```python
from build123d import *

# Parameters (mm, degrees)
SKETCH1_W           = 1000
SKETCH1_H           = 500
BOSS_EXTRUDE1_DEPTH = 400
SKETCH2_R           = 150
BOSS_EXTRUDE2_DEPTH = 150


with BuildPart() as part:
    # Sketch1 → Boss-Extrude1 (new body)
    with BuildSketch(Plane(origin=(0, 0, 0), x_dir=(1, 0, 0), z_dir=(0, 1, 0))):
        Polygon((1400, -200), (1000, 0), (1000, 500), (1400, 700), align=None)
        with Locations((500, 250)):
            Rectangle(SKETCH1_W, SKETCH1_H)
    extrude(amount=BOSS_EXTRUDE1_DEPTH)

    # Sketch2 → Boss-Extrude2 (add)
    with BuildSketch(Plane(origin=(0, 400, 0), x_dir=(1, 0, 0), z_dir=(0, 1, 0))):
        with Locations(Location((500, 250, 0), (0, 0, 270))):
            Circle(SKETCH2_R)
    extrude(amount=BOSS_EXTRUDE2_DEPTH)


solid = part.part
```
Source: CAD feature listing. Evaluate the final solid. Frame: model axes, mm. A direction names the side the tool comes from. Round coordinates to 2 decimals unless told otherwise and drop trailing zeros. Order: outer loops, then holes, each group sorted by start corner. A loop starts at its lowest first (then second) coordinate and runs counter-clockwise, first axis right, second up. Notation, with made-up numbers: (30, 6) -> (45, 6) arc R8 cw to (45, 10) -> close; hole circle Ø4 at (0, -34). An arc over 180 degrees is marked (long way). Use CSV: the item, a comma, the result in double quotes.
(1) Section C-C on y = 137.5. Return the cut outline in (x, z).
Report:
outline,"(0, -500) -> (1000, -500) -> (1400, -700) -> (1400, 200) -> (1000, 0) -> (0, 0) -> close"
(2) Section A-A on z = -250. Return the cut outline in (x, y).
Report:
outline,"(0, 0) -> (1400, 0) -> (1400, 400) -> (650, 400) -> (650, 550) -> (350, 550) -> (350, 400) -> (0, 400) -> close"
(3) Access query for faces 1 (the face through (710, 0, -256)), 2 (the face through (493, 197, 0)), 3 (the face through (493, 197, -500)), 4 (the face through (502, 550, -252)), 5 (the face through (545.06, 473.95, -106.93)). Directions: +Z, -Z, +X, -X, +Y, -Y. A direction counts if a zero-diameter tool reaches every point of the face in a straight line with its end or side. Return the directions, or none.
Report:
face 1,"+Z, -Z, +X, -X, -Y"
face 2,"+Z, -X, +Y, -Y"
face 3,"-Z, -X, +Y, -Y"
face 4,"+Z, -Z, +X, -X, +Y"
face 5,"+Y"
(4) Ray query, L1, parallel to Z at x = 220.5, y = 146; L2, parallel to Y at x = 222.5, z = -35.5; L3, parallel to X at y = 119, z = 150.5. Return the intervals inside material, ascending.
Report:
L1,"-500 to 0"
L2,"0 to 400"
L3,"1301 to 1400"
(5) Section D-D on z = -593.5. Return the cut outline in (x, y), and give its area (3 significant figures).
Report:
outline,"(1187, 0) -> (1400, 0) -> (1400, 400) -> (1187, 400) -> close"
area,"85,200 mm^2"
(6) First-contact query: pin 1 Ø4 at (x, y) = (620, 127) entering from +Z; pin 2 Ø2 at (x, z) = (912.5, -449) entering from +Y; pin 3 Ø10 at (x, y) = (435.5, 296.5) entering from -Z. Flat tips, straight axial feed; report the tip coordinate or a pass-through.
Report:
pin 1,"z = 0"
pin 2,"y = 400"
pin 3,"z = -500"
(7) Section B-B on x = 500. Return the cut outline in (y, z).
Report:
outline,"(0, -500) -> (400, -500) -> (400, -400) -> (550, -400) -> (550, -100) -> (400, -100) -> (400, 0) -> (0, 0) -> close"
